from build123d import *

# Parameters (mm, degrees)
ESQUISSE1_R             = 5
BASE_EXTRUSION_DEPTH    = 9.5
ESQUISSE2_R             = 2.5
BOSS_EXTRU_1_DEPTH      = 5
CONG_1_R                = 0.5
ENL_V_MAT_EXTRU_1_DEPTH = 16
ESQUISSE11_R            = 2
BOSS_EXTRU_2_DEPTH      = 1.5
BOSS_EXTRU_3_DEPTH      = 6
ESQUISSE13_R            = 1
ENL_V_MAT_EXTRU_2_DEPTH = 18
CHANFREIN1_SIZE         = 0.25


with BuildPart() as part:
    # Esquisse1 → Base-Extrusion (new body)
    with BuildSketch(Plane.XY):
        Circle(ESQUISSE1_R)
    extrude(amount=BASE_EXTRUSION_DEPTH)

    # Esquisse2 → Boss.-Extru.1 (add)
    with BuildSketch(Plane.XY.offset(9.5)):
        Circle(ESQUISSE2_R)
    extrude(amount=BOSS_EXTRU_1_DEPTH)

    # Congé1
    cong_1_edges = [part.edges().sort_by_distance(p)[0] for p in [
        (-5, 0, 9.5),
    ]]
    fillet(cong_1_edges, radius=CONG_1_R)

    # Esquisse7 → Enlèv. mat.-Extru.1 (cut, symmetric)
    with BuildSketch(Plane(origin=(0, 0, 0), x_dir=(0, 0, -1), z_dir=(1, 0, 0))):
        with BuildLine():
            Line((1, 1.25), (-7, 1.25))
            ThreePointArc((-7, 1.25), (-8.25, 0), (-7, -1.25))
            Line((-7, -1.25), (1, -1.25))
            Line((1, -1.25), (1, 1.25))
        make_face()
    extrude(amount=ENL_V_MAT_EXTRU_1_DEPTH, both=True, mode=Mode.SUBTRACT)

    # Esquisse8 → Enlèvement de matière-Révolution1 (revolve, cut)
    with BuildSketch(Plane(origin=(0, 0, 0), x_dir=(0, 0, -1), z_dir=(1, 0, 0))):
        Polygon((0, 4.5), (-4, 3), (-8, 3), (-9.5, 0), (0, 0), align=None)
    revolve(axis=Axis((0, 0, 0), (0, 0, 1)), mode=Mode.SUBTRACT)

    # Esquisse11 → Boss.-Extru.2 (add)
    with BuildSketch(Plane.XY.offset(14.5)):
        Circle(ESQUISSE11_R)
    extrude(amount=BOSS_EXTRU_2_DEPTH)

    # Esquisse12 → Boss.-Extru.3 (add)
    with BuildSketch(Plane.XY.offset(16)):
        Polygon((-0.124297896, 2.371745145), (0, 2.5), (0.124297896, 2.371745145), (0.261321158, 2.486304738), (0.371531854, 2.345759809), (0.519779227, 2.445369002), (0.614695232, 2.294073837), (0.772542486, 2.377641291), (0.85112388, 2.217253513), (1.016841608, 2.283863644), (1.078227437, 2.116140495), (1.25, 2.165063509), (1.293517708, 1.991842599), (1.469463131, 2.022542486), (1.494635929, 1.845721658), (1.672826516, 1.857862064), (1.679378605, 1.679378605), (1.857862064, 1.672826516), (1.845721658, 1.494635929), (2.022542486, 1.469463131), (1.991842599, 1.293517708), (2.165063509, 1.25), (2.116140495, 1.078227437), (2.283863644, 1.016841608), (2.217253513, 0.85112388), (2.377641291, 0.772542486), (2.294073837, 0.614695232), (2.445369002, 0.519779227), (2.345759809, 0.371531854), (2.486304738, 0.261321158), (2.371745145, 0.124297896), (2.5, 0), (2.371745145, -0.124297896), (2.486304738, -0.261321158), (2.345759809, -0.371531854), (2.445369002, -0.519779227), (2.294073837, -0.614695232), (2.377641291, -0.772542486), (2.217253513, -0.85112388), (2.283863644, -1.016841608), (2.116140495, -1.078227437), (2.165063509, -1.25), (1.991842599, -1.293517708), (2.022542486, -1.469463131), (1.845721658, -1.494635929), (1.857862064, -1.672826516), (1.679378605, -1.679378605), (1.672826516, -1.857862064), (1.494635929, -1.845721658), (1.469463131, -2.022542486), (1.293517708, -1.991842599), (1.25, -2.165063509), (1.078227437, -2.116140495), (1.016841608, -2.283863644), (0.85112388, -2.217253513), (0.772542486, -2.377641291), (0.614695232, -2.294073837), (0.519779227, -2.445369002), (0.371531854, -2.345759809), (0.261321158, -2.486304738), (0.124297896, -2.371745145), (0, -2.5), (-0.124297896, -2.371745145), (-0.261321158, -2.486304738), (-0.371531854, -2.345759809), (-0.519779227, -2.445369002), (-0.614695232, -2.294073837), (-0.772542486, -2.377641291), (-0.85112388, -2.217253513), (-1.016841608, -2.283863644), (-1.078227437, -2.116140495), (-1.25, -2.165063509), (-1.293517708, -1.991842599), (-1.469463131, -2.022542486), (-1.494635929, -1.845721658), (-1.672826516, -1.857862064), (-1.679378605, -1.679378605), (-1.857862064, -1.672826516), (-1.845721658, -1.494635929), (-2.022542486, -1.469463131), (-1.991842599, -1.293517708), (-2.165063509, -1.25), (-2.116140495, -1.078227437), (-2.283863644, -1.016841608), (-2.217253513, -0.85112388), (-2.377641291, -0.772542486), (-2.294073837, -0.614695232), (-2.445369002, -0.519779227), (-2.345759809, -0.371531854), (-2.486304738, -0.261321158), (-2.371745145, -0.124297896), (-2.5, 0), (-2.371745145, 0.124297896), (-2.486304738, 0.261321158), (-2.345759809, 0.371531854), (-2.445369002, 0.519779227), (-2.294073837, 0.614695232), (-2.377641291, 0.772542486), (-2.217253513, 0.85112388), (-2.283863644, 1.016841608), (-2.116140495, 1.078227437), (-2.165063509, 1.25), (-1.991842599, 1.293517708), (-2.022542486, 1.469463131), (-1.845721658, 1.494635929), (-1.857862064, 1.672826516), (-1.679378605, 1.679378605), (-1.672826516, 1.857862064), (-1.494635929, 1.845721658), (-1.469463131, 2.022542486), (-1.293517708, 1.991842599), (-1.25, 2.165063509), (-1.078227437, 2.116140495), (-1.016841608, 2.283863644), (-0.85112388, 2.217253513), (-0.772542486, 2.377641291), (-0.614695232, 2.294073837), (-0.519779227, 2.445369002), (-0.371531854, 2.345759809), (-0.261321158, 2.486304738), align=None)
    extrude(amount=BOSS_EXTRU_3_DEPTH)

    # Esquisse13 → Enlèv. mat.-Extru.2 (cut)
    with BuildSketch(Plane.XY.offset(22)):
        Circle(ESQUISSE13_R)
    extrude(amount=-ENL_V_MAT_EXTRU_2_DEPTH, mode=Mode.SUBTRACT)

    # Chanfrein1
    chanfrein1_edges = [part.edges().sort_by_distance(p)[0] for p in [
        (-1, 0, 22),
        (-2.5, 0, 14.5),
    ]]
    chamfer(chanfrein1_edges, length=CHANFREIN1_SIZE)


solid = part.part
Model file for the job. Use its own axes, mm. A direction names the side the tool comes from. Give positions to 0.01 mm unless a question says otherwise; leave off trailing zeros. Order: outer loops, then holes, each group sorted by start corner. A loop starts at its lowest first (then second) coordinate and runs counter-clockwise, first axis right, second up. Notation, with made-up numbers: (11.5, 8.25) - (39.5, 8.25) arc R26 ccw to (39.5, 34.25) - close; hole circle Ø1 at (12.5, 86). An arc over 180 degrees is marked (long way). Return JSON: item names as keys, results as strings.
1) Probe line 1 (Y direction, x = 2, z = 6.75); line 2 (Y direction, x = 3.5, z = 5.5); line 3 (Z direction, x = -1.75, y = 1.5). List the from-to ranges inside material, lowest first. Write a range as from..to.
Geometry says:
{"line 1": "-4.58..-2.24, 2.24..4.58", "line 2": "-3.57..-1.25, 1.25..3.57", "line 3": "8.35..14.45, 16..22"}
2) Cut at A-A, the plane z = 5.5. Give the cut face in (x, y), plus the area to 3 significant figures.
Geometry says:
{"outline": "(-4.84, -1.25) arc R5 ccw to (4.84, -1.25) - (2.73, -1.25) arc R3 cw to (-2.73, -1.25) - close; (-4.84, 1.25) - (-2.73, 1.25) arc R3 cw to (2.73, 1.25) - (4.84, 1.25) arc R5 ccw to start", "area": "40.1 mm²"}
3) 3-axis set-ups, long thin cutter, end or side, ignore diameter. For faces 4 (the cylindrical face through (0, -1, 15)), 5 (the flat face through (2, -2, 9.5)), 6 (the flat face through (0, 4.7, 0)), 7 (the flat face through (4, -1.25, 4)), 8 (the cylindrical face through (0, -3, 6)): which of +Z, -Z, +X, -X, +Y, -Y reach the whole face in a straight line?
Geometry says:
{"face 4": "+Z, -Z", "face 5": "+Z", "face 6": "-Z, +X, -X, +Y, -Y", "face 7": "-Z, +X, -X", "face 8": "-Z"}
4) Flat gauge pins, fed straight in: P1, Ø1.1, axis at x = 3.5, z = 4, coming from the -Y side; P2, Ø1.5, axis at y = 0.5, z = 10, coming from the -X side; P3, Ø4, axis at x = 1, y = 0, coming from the -Z side; P4, Ø1.8, axis at x = 0, y = 0, coming from the +Z side. Where does each tip first touch, or does it go through?
Geometry says:
{"P1": "y = -4.04", "P2": "x = -4.91", "P3": "z = 8.02", "P4": "through"}
5) Cut at B-B, the plane z = 15. Give the cut face in (x, y).
Geometry says:
{"outline": "circle Ø4 at (0, 0); hole circle Ø2 at (0, 0)"}
6) Cut at C-C, the plane z = 8.75. Give the cut face in (x, y), plus the area to 3 significant figures.
Geometry says:
{"outline": "circle Ø10 at (0, 0); hole circle Ø3 at (0, 0)", "area": "71.5 mm²"}
7) Pull direction X, two halves, no side cores. Call faces 1 (the cylindrical face through (0, -2, 15)), 2 (the flat face through (-0.38, -4.64, 0)), 3 (the conical face through (-0.064, -3.572, 2.472)): pulls with the +X half, pulls with the -X half, needs draft (parallel to the pull), parting line crosses it, or undercut.
Geometry says:
{"face 1": "parting line crosses it", "face 2": "needs draft", "face 3": "undercut"}
